Can you work these out from the model? Positions are in its coordinate system, mm. A direction names the side the tool comes from. Round coordinates to 2 decimals unless told otherwise and drop trailing zeros. Write each loop counter-clockwise with the first axis right and the second up, starting at its lowest first coordinate (ties: lowest second). Pieces come first, ordered by that corner, then holes.
Q1. If we section it at D-D (z = 1.85): Please give me the cut outline in (x, y), plus the area to 3 significant figures.
Q2. We'd pull the mould along X, two halves only. Please class faces 4 (the cylindrical face through (0.434, -1.952, 0.246)), 5 (the flat face through (-2, 2, 3.5)), 6 (the cylindrical face through (-0.867, 3.905, 1.923)): +X half, -X half, draft (parallel to the pull), parting line (faces both ways), or undercut.
Q3. I'm going to push flat-ended pins straight in: pin 1 Ø1.5 at (y, z) = (3, 3) entering from -X; pin 2 Ø1 at (x, z) = (2.5, 0.5) entering from -Y; pin 3 Ø1.8 at (x, y) = (0, 0) entering from +Z. Where does each tip first touch, or does it pass through?
Q4. Please list where these lines run through material, in increasing order: line 1 along Y through (x, z) = (0, 3.65); line 2 along X through (y, z) = (-1.75, 0.65); line 3 along Y through (x, z) = (-0.75, 3.7).
Q5. If we section it at C-C (z = 3.6): Please give me the cut outline in (x, y), plus the area to 3 significant figures.
Q6. For faces 1 (the cylindrical face through (0.434, 1.952, 3.703)), 2 (the cylindrical face through (-1.5, -0.07, 1.92)), 3 (the cylindrical face through (-3.233, 1.341, 0.254)), which set-ups out of +Z, -Z, +X, -X, +Y, -Y let a thin tool reach every point of the face, with its end or its side?
Solid Edge part; units mm, degrees
sketch "Sketch1" plane through (0, 0, 0) normal (0, 0, 1) x (1, 0, 0)
  circle A0 centre (0, 0) radius 1.5
  circle A1 centre (0, 0) radius 4
extrude "Protrusion1" add sketch "Sketch1" along normal blind 4
sketch "Sketch2" plane through (0, 0, 0) normal (0, -1, 0) x (1, 0, 0)
  line L0 (-3.5, 4) -> (-2, 4)
  line L1 (-2, 3.5) -> (-2, 4)
  line L2 (-3.5, 3.5) -> (-2, 3.5)
  line L3 (-3.5, 4) -> (-3.5, 3.5)
  line L4 (-3.5, 0) -> (-2, 0)
  line L5 (-2, 0.5) -> (-2, 0)
  line L6 (-3.5, 0.5) -> (-2, 0.5)
  line L7 (-3.5, 0) -> (-3.5, 0.5)
revolve "RevolvedCutout1" cut sketch "Sketch2" angle 360 about axis through (0, 0, 0) along (0, 0, 1)
fillet "Round_1" radius 0.1 4 edges at (2, 0, 4) (-1.5, 0, 4) (3.5, 0, 4) (-4, 0, 4)
A:
1. outline: circle Ø8 at (0, 0); hole circle Ø3 at (0, 0)
1. area: 43.2 mm2
2. face 4: undercut
2. face 5: undercut
2. face 6: parting line
3. pin 1: stops at x = -3.31
3. pin 2: stops at y = -3.46
3. pin 3: passes through
4. line 1: y = -4 to -3.5, -2 to -1.5, 1.5 to 2, 3.5 to 4
4. line 2: x = -3.6 to 3.6
4. line 3: y = -3.93 to -3.42, -1.85 to -1.3, 1.3 to 1.85, 3.42 to 3.93
5. outline: circle Ø8 at (0, 0); circle Ø4 at (0, 0); hole circle Ø7 at (0, 0); hole circle Ø3 at (0, 0)
5. area: 17.3 mm2
6. face 1: +Z
6. face 2: +Z, -Z
6. face 3: -Z
